Here's how the part is built. I have some questions about the finished solid (model axes, mm). A direction names the side the tool comes from. Round coordinates to 2 decimals unless told otherwise and drop trailing zeros. Loops run counter-clockwise (first coordinate to the right, second up) from the corner with the lowest first, then second, coordinate; pieces in that order, holes last. Notation, with made-up numbers: (-38.75, 32.5) - (-2.75, 32.5) arc R13 ccw to (-2.75, 57.5) - close; hole circle Ø2 at (11, 11.25). An arc over 180 degrees is marked (long way). Answer as a JSON object with one key per item and string values. Group by question number.
1) I want a section at C-C, the plane y = -13.5. Please give me the cut outline in (x, z).
2) I want a section at A-A, the plane x = -20.5. Please give me the cut outline in (y, z), then the cut area to 3 significant figures.
3) I want a section at B-B, the plane z = 6. Give the number of separate pieces and of enclosed holes in the cut face, then the cut area to 3 significant figures.
4) I want a section at D-D, the plane x = 22.5. Please give me the cut outline in (y, z).
5) If we mould it in two halves opening along Y, with no side actions, what happens to faces 1 (the face through (29.94, -1.91, 6.26)), 2 (the face through (-18.71, -6.31, 6.26)), 3 (the face through (-31.75, -9, 6))? For each: pulls with the +Y half, pulls with the -Y half, needs draft (parallel to the pull), parting line crosses it, or undercut.
6) If I drill on line 1 along X through (y, z) = (-5.75, 2.75); line 2 along X through (y, z) = (-9.25, 7.5); line 3 along X through (y, z) = (-1.5, 18), over which ranges is the centre line in solid material (lowest first)? Write a range as [from, to].
7) Will these pins go through, and if not, where does the flat tip stop? P1, Ø4, axis at x = -28, y = -12, coming from the +Z side; P2, Ø1, axis at x = 18, z = 15, coming from the +Y side; P3, Ø2.5, axis at y = -7, z = 21.5, coming from the -X side; P4, Ø8.5, axis at y = -7, z = 20, coming from the +X side.
8) Which directions (+Z, -Z, +X, -X, +Y, -Y) give clear straight access to the entire face, cutting with the end or side of a thin tool? Please do faces 4 (the face through (-12.7, -9, 22)), 5 (the face through (12.7, -9, 22)), 6 (the face through (17.467, -9.316, 6.261)).
from build123d import *

# Parameters (mm, degrees)
F1_DEPTH = 19.05
F3_D     = 9.525
F4_R     = 6.35
F6_R     = 5.08


with BuildPart() as f1:
    # F0 (on Front) → F1 (new body)
    with BuildSketch(Plane.XZ):
        Polygon((-31.75, 0), (0, 0), (0, 25.4), (-12.7, 25.4), (-12.7, 12.7), (-31.75, 12.7), align=None)
    extrude(amount=F1_DEPTH)

    # F3 (through all)
    with Locations(Plane.XY.offset(12.7)):
        with Locations((-22.225, -9.525)):
            Hole(F3_D / 2)

    # F4
    f4_edges = [f1.edges().sort_by_distance(p)[0] for p in [
        (-31.75, -19.05, 6.35),
        (-31.75, 0, 6.35),
    ]]
    fillet(f4_edges, radius=F4_R)

    # F5: F1 across face


with BuildPart() as f1_1:
    add(f1.part)
    add(f1.part.mirror(Plane(origin=(0, -9.525, 12.7), x_dir=(0, 1, 0), z_dir=(1, 0, 0))))

    # F6
    f6_edges = [f1_1.edges().sort_by_distance(p)[0] for p in [
        (-12.7, -9.525, 12.7),
        (12.7, -9.525, 12.7),
    ]]
    fillet(f6_edges, radius=F6_R)


solid = f1_1.part
Outcome:
{
 "1": {"outline": "(-31.7, 0) - (-24.85, 0) - (-24.85, 12.7) - (-31.7, 12.7) - close; (-19.6, 0) - (19.6, 0) - (19.6, 12.7) - (17.78, 12.7) arc R5.08 cw to (12.7, 17.78) - (12.7, 25.4) - (-12.7, 25.4) - (-12.7, 17.78) arc R5.08 cw to (-17.78, 12.7) - (-19.6, 12.7) - close; (24.85, 0) - (31.7, 0) - (31.7, 12.7) - (24.85, 12.7) - close"},
 "2": {"outline": "(-19.05, 0) - (-13.96, 0) - (-13.96, 12.7) - (-19.05, 12.7) - close; (-5.09, 0) - (0, 0) - (0, 12.7) - (-5.09, 12.7) - close", "area": "129 mm^2"},
 "3": {"separate pieces": "1", "enclosed holes": "2", "area": "1,030 mm^2"},
 "4": {"outline": "(-19.05, 0) - (-14.28, 0) - (-14.28, 12.7) - (-19.05, 12.7) - close; (-4.77, 0) - (0, 0) - (0, 12.7) - (-4.77, 12.7) - close"},
 "5": {"face 1": "pulls with the +Y half", "face 2": "undercut", "face 3": "needs draft"},
 "6": {"line 1": "[-31.72, -25.13], [-19.32, 19.32], [25.13, 31.72]", "line 2": "[-31.75, -26.98], [-17.47, 17.47], [26.98, 31.75]", "line 3": "[-12.7, 12.7]"},
 "7": {"P1": "z = 12.7", "P2": "through", "P3": "x = -12.7", "P4": "x = 13.12"},
 "8": {"face 4": "+Z, -X, +Y, -Y", "face 5": "+Z, +X, +Y, -Y", "face 6": "+Z, -Z"}
}
